CAD build for the part. Positions are in the model's coordinates, mm. Face numbers are marked on the shaded views. Coordinates: 2 decimals unless noted, no trailing zeros. Order: outer loops, then holes, each group sorted by start corner. A loop starts at its lowest first (then second) coordinate and runs counter-clockwise, first axis right, second up. Notation, with made-up numbers: M -38.75,32 L -12.75,32 A8 cw -12.75,42 Z; hole C 64.25,15 d4. An arc over 180 degrees is marked long. One line per item, written item: value.
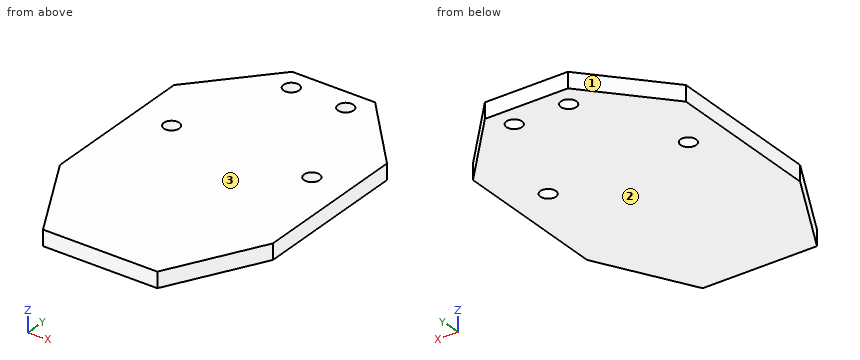
from build123d import *

# Parameters (mm, degrees)
SKETCH_1_R      = 1.5
EXTRUDE_1_DEPTH = 3


with BuildPart() as part:
    # 草图1 → 凸台-拉伸1 (new body)
    with BuildSketch(Plane.XY):
        Polygon((11, 0), (-11, 0), (-20.5, 17.599715907), (-20.5, 47.899715907), (-7.989824602, 62), (7.989824602, 62), (20.5, 47.899715907), (20.5, 17.599715907), align=None)
        with Locations((-5.239824602, 58)):
            Circle(SKETCH_1_R, mode=Mode.SUBTRACT)
        with Locations((-13.5, 37.599715907)):
            Circle(SKETCH_1_R, mode=Mode.SUBTRACT)
        with Locations((13.5, 37.599715907)):
            Circle(SKETCH_1_R, mode=Mode.SUBTRACT)
        with Locations((5.239824602, 58)):
            Circle(SKETCH_1_R, mode=Mode.SUBTRACT)
    extrude(amount=EXTRUDE_1_DEPTH)


solid = part.part
Q1. Drill centre lines: line 1 along Y through (x, z) = (5.5, 2.6); line 2 along Y through (x, z) = (-13.5, 2); line 3 along X through (y, z) = (9, 2). Where is each one in solid material? Low to high.
Recorded:
line 1: y = 0 to 56.52, 59.48 to 62
line 2: y = 4.63 to 36.1, 39.1 to 55.79
line 3: x = -15.86 to 15.86
Q2. Mould opens along Z. For the marked faces 1, 2 and 3 say: released by +Z, released by -Z, zero draft, split by the parting line, or undercut.
Recorded:
face 1: zero draft
face 2: released by -Z
face 3: released by +Z
Q3. Slice it at B-B (x = -13.5). List the corners of the cut face in (y, z), plus the area to 3 significant figures.
Recorded:
outline: M 4.63,0 L 36.1,0 L 36.1,3 L 4.63,3 Z; M 39.1,0 L 55.79,0 L 55.79,3 L 39.1,3 Z
area: 144 mm^2
Q4. Slice it at A-A (z = 2.5). List the corners of the cut face in (x, y), plus the area to 3 significant figures.
Recorded:
outline: M -20.5,17.6 L -11,0 L 11,0 L 20.5,17.6 L 20.5,47.9 L 7.99,62 L -7.99,62 L -20.5,47.9 Z; hole C -13.5,37.6 d3; hole C -5.24,58 d3; hole C 5.24,58 d3; hole C 13.5,37.6 d3
area: 2,170 mm^2
Q5. Slice it at D-D (x = 5.5). List the corners of the cut face in (y, z).
Recorded:
outline: M 0,0 L 56.52,0 L 56.52,3 L 0,3 Z; M 59.48,0 L 62,0 L 62,3 L 59.48,3 Z
Q6. Slice it at C-C (y = 58). List the corners of the cut face in (x, z).
Recorded:
outline: M -11.54,0 L -6.74,0 L -6.74,3 L -11.54,3 Z; M -3.74,0 L 3.74,0 L 3.74,3 L -3.74,3 Z; M 6.74,0 L 11.54,0 L 11.54,3 L 6.74,3 Z
